```python
from build123d import *

# Parameters (mm, degrees)
F0_W     = 118.7662929296
F0_H     = 88.2422402501
F1_DEPTH = 50
F3_D     = 16.75
F5_D     = 30
F6_T     = -2.54


with BuildPart() as f1:
    # F0 (on Top) → F1 (new body)
    with BuildSketch(Plane.XY):
        with Locations((-3.1449049711, 3.6998838186)):
            Rectangle(F0_W, F0_H)
    extrude(amount=F1_DEPTH)

    # F3 (through all)
    with Locations(Plane.XY.offset(50)):
        with Locations((-41.7324155569, 28.2360911369), (27.3362733424, 28.2360911369), (28.1245876104, -22.8877589107), (-41.7324155569, -22.4902890623)):
            Hole(F3_D / 2)

    # F5 (through all)
    with Locations(Plane.XZ.offset(40.4212363064)):
        with Locations((-2.2715097293, 25.5605392158)):
            Hole(F5_D / 2)

    # F6
    f6_openings = [f1.faces().sort_by_distance(p)[0] for p in [
        (56.238241, 3.699884, 25),
        (-62.528051, 3.699884, 25),
    ]]
    offset(amount=F6_T, openings=f6_openings)


solid = f1.part
```
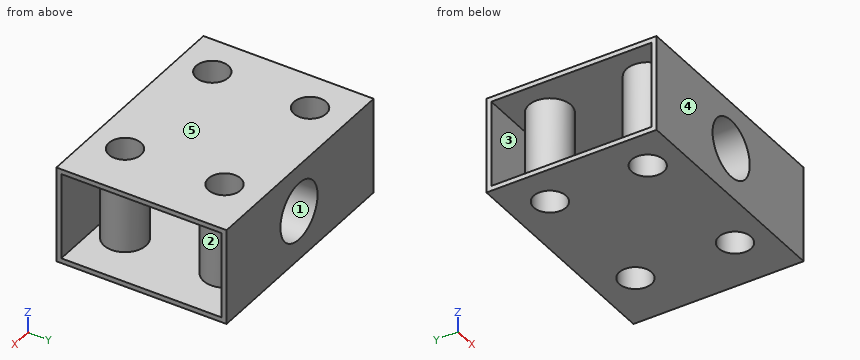
Could you check a few things on this model? Use its own coordinates, in mm. Face numbers are marked on the shaded views. A direction names the side the tool comes from. Round coordinates to 2 decimals unless told otherwise and drop trailing zeros. Loops run counter-clockwise (first coordinate to the right, second up) from the corner with the lowest first, then second, coordinate; pieces in that order, holes last.
Q1. I want a section at C-C (x = 41). Write out the boundary of the cut face in (y, z).
Q2. Please list where these lines run through material, in increasing order: L1, parallel to Y at x = 28, z = 14; L2, parallel to Z at x = -28, y = 21; L3, parallel to X at y = -23, z = 14.
Q3. Thinking about a two-plate mould opening in Y: for the marked faces 3, 4 and 5, which applies, pulls with the +Y half, pulls with the -Y half, needs draft (parallel to the pull), parting line crosses it, or undercut?
Q4. I want a section at D-D (y = 14.5). Write out the boundary of the cut face in (x, z).
Q5. On a 3-axis mill with a long thin cutter (end or side, diameter ignored), from which of +Z, -Z, +X, -X, +Y, -Y can I reach the whole of each face in a straight line? I mean the marked faces 1 and 2. Say none if no direction works.
Q6. I want a section at B-B (z = 19.5). Give the number of separate pieces and of enclosed holes in the cut face, and give its area (3 significant figures).
Q7. I want a section at A-A (x = 22.5). Write out the boundary of the cut face in (y, z).
Answer below:
1. outline: (-40.42, 0) - (47.82, 0) - (47.82, 50) - (-40.42, 50) - close; hole (-37.88, 2.54) - (45.28, 2.54) - (45.28, 47.46) - (-37.88, 47.46) - close
2. L1: y = -40.42 to -37.88, -33.8 to -31.26, -14.51 to -11.97, 17.34 to 19.89, 36.58 to 39.13, 45.28 to 47.82
2. L2: z = 0 to 2.54, 47.46 to 50
2. L3: x = -52.64 to -50.09, -33.37 to -30.83, -15.46 to -11.83, 7.29 to 10.92, 17.21 to 19.75, 36.5 to 39.04
3. face 3: undercut
3. face 4: pulls with the -Y half
3. face 5: needs draft
4. outline: (-62.53, 0) - (56.24, 0) - (56.24, 2.54) - (-62.53, 2.54) - close; (-62.53, 47.46) - (56.24, 47.46) - (56.24, 50) - (-62.53, 50) - close; circle Ø35.08 at (-2.27, 25.56); hole circle Ø30 at (-2.27, 25.56)
5. face 1: +Y, -Y
5. face 2: none
6. separate pieces: 6
6. enclosed holes: 4
6. area: 1,540 mm2
7. outline: (-40.42, 0) - (-29.09, 0) - (-29.09, 50) - (-40.42, 50) - close; (-16.68, 0) - (21.4, 0) - (21.4, 50) - (-16.68, 50) - close; (35.07, 0) - (47.82, 0) - (47.82, 50) - (35.07, 50) - close; hole (-37.88, 2.54) - (-32.24, 2.54) - (-32.24, 47.46) - (-37.88, 47.46) - close; hole (-13.53, 2.54) - (18.45, 2.54) - (18.45, 47.46) - (-13.53, 47.46) - close; hole (38.02, 2.54) - (45.28, 2.54) - (45.28, 47.46) - (38.02, 47.46) - close
